```python
from build123d import *

# Parameters (mm, degrees)
F0_R      = 120.65
F1_DEPTH  = 3.175
F2_R      = 119.0625
F3_DEPTH  = 9.525
F4_SIZE2  = 9.52499
F4_SIZE   = 3.17499
F5_R      = 2.38125
F6_DEPTH  = 101.6
F7_R      = 119.0625
F8_DEPTH  = 9.525
F9_R      = 120.65
F10_DEPTH = 3.175
F11_SIZE2 = 3.17499
F11_SIZE  = 9.52499
F12_R     = 12.7
F13_DEPTH = 127.001


# Not quite as in the source:
# - a fillet or chamfer is up to 0.001 mm smaller than in the source, because OpenCascade refuses the exact size


with BuildPart() as f1:
    # F0 (on Right) → F1 (new body)
    with BuildSketch(Plane.YZ):
        Circle(F0_R)
    extrude(amount=F1_DEPTH)

    # F2 (on face) → F3 (join)
    with BuildSketch(Plane.YZ.offset(3.175)):
        Circle(F2_R)
    extrude(amount=F3_DEPTH)

    # F4 (size 3.175 and 9.525 in the source; OpenCascade refuses exactly that, so slightly less here)
    f4_edges = [f1.edges().sort_by_distance(p)[0] for p in [
        (12.7, -119.0625, 0),
    ]]
    f4_side = f1.faces().sort_by_distance((12.7, 0, 0))[0]
    chamfer(f4_edges, length=F4_SIZE, length2=F4_SIZE2, reference=f4_side)

    # F5 (on face) → F6 (join)
    with BuildSketch(Plane.YZ.offset(12.7)):
        with BuildLine():
            ThreePointArc((21.1539941395, 14.0594641416), (-24.3153393061, -7.3433149482), (25.4, 0))
            ThreePointArc((25.4, 0), (24.3153393061, 7.3433149482), (21.1539941395, 14.0594641416))
        make_face()
        with Locations((0, -76.2)):
            Circle(F5_R)
        with Locations((65.9911357684, 38.1)):
            Circle(F5_R)
        with Locations((-65.9911357684, 38.1)):
            Circle(F5_R)
    extrude(amount=F6_DEPTH)

    # F7 (on face) → F8 (join)
    with BuildSketch(Plane.YZ.offset(114.3)):
        Circle(F7_R)
    extrude(amount=F8_DEPTH)

    # F9 (on face) → F10 (join)
    with BuildSketch(Plane.YZ.offset(123.825)):
        Circle(F9_R)
    extrude(amount=F10_DEPTH)

    # F11 (size 9.525 and 3.175 in the source; OpenCascade refuses exactly that, so slightly less here)
    f11_edges = [f1.edges().sort_by_distance(p)[0] for p in [
        (114.3, -119.0625, 0),
    ]]
    f11_side = f1.faces().sort_by_distance((119.0625, -119.0625, 0))[0]
    chamfer(f11_edges, length=F11_SIZE, length2=F11_SIZE2, reference=f11_side)

    # F12 (on face) → F13 (cut, through all)
    with BuildSketch(Plane.YZ.offset(127)):
        Circle(F12_R)
    extrude(amount=-F13_DEPTH, mode=Mode.SUBTRACT)


solid = f1.part
```
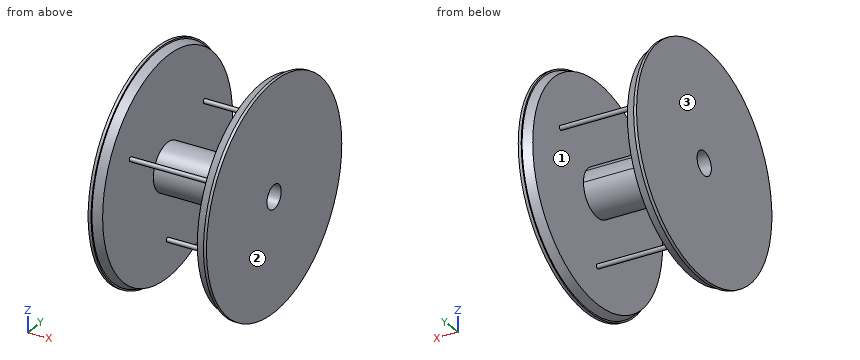
Can you work these out from the model? Positions are in its coordinate system, mm. Face numbers are marked on the shaded views. Give positions to 0.01 mm unless a question says otherwise; leave off trailing zeros. Loops run counter-clockwise (first coordinate to the right, second up) from the corner with the lowest first, then second, coordinate; pieces in that order, holes last. Notation, with made-up numbers: M 84.5,-3.5 L 94.5,-3.5 A12 cw 94.5,8.5 Z; hole C 3.5,-36.75 d10. An arc over 180 degrees is marked long. One line per question, with ' | ' between items. Start each with the question number.
Q1. For pin 1 Ø1.5 at (x, y) = (112.5, 45) entering from -Z; pin 2 Ø4 at (x, y) = (112, -2) entering from -Z; pin 3 Ø12 at (x, z) = (61, -81.5) entering from +Y, each with a flat end and sliding along its axis, tell me the tip position at first contact or that it passes through.
Q2. If we section it at A-A (x = 44.5): Please give me the cut outline in (y, z).
Q3. If we mould it in two halves opening along X, with no side actions, what happens to the marked faces 1, 2 and 3? For each: +X half, -X half, draft (parallel to the pull), parting line (faces both ways), or undercut.
Q4. If I drill on line 1 (Z direction, x = 31, y = 0); line 2 (X direction, y = 57, z = -69.5); line 3 (Y direction, x = 39.5, z = -5), over which ranges is the centre line in solid material (lowest first)? Write a range as from..to.
Computed:
1) pin 1: passes through | pin 2: stops at z = -78.58 | pin 3: stops at y = 2.38
2) outline: C -65.99,38.1 d4.76; C 0,0 d50.8; C 0,-76.2 d4.76; C 65.99,38.1 d4.76; hole C 0,0 d25.4
3) face 1: undercut | face 2: +X half | face 3: -X half
4) line 1: z = -78.58..-73.82, -25.4..-12.7, 12.7..25.4 | line 2: x = 0..12.7, 114.3..127 | line 3: y = -24.9..-11.67, 11.67..24.9
